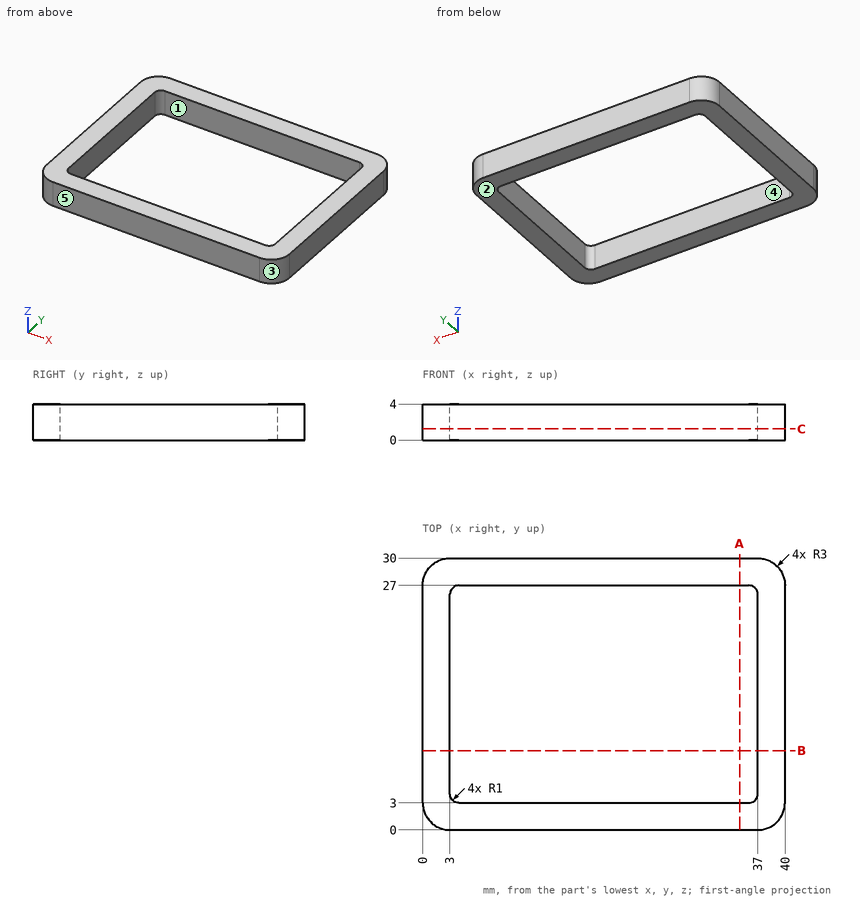
Geometry check sheet. Reference: drawing and pictorial views, mm from the part's lowest x, y, z. A direction names the side the tool comes from. Round coordinates to 2 decimals unless told otherwise and drop trailing zeros. Loops run counter-clockwise (first coordinate to the right, second up) from the corner with the lowest first, then second, coordinate; pieces in that order, holes last. Notation, with made-up numbers: (47.5, 12) -> (62.5, 12) arc R18 ccw to (62.5, 44) -> close; hole circle Ø6 at (58, 2.5). An arc over 180 degrees is marked (long way). Answer as a JSON object with one key per item and string values. Group by question number.
Item 1: Release check for a two-part mould opening along Y. For the marked faces 1, 2 and 3 record: pulls with the +Y half, pulls with the -Y half, needs draft (parallel to the pull), parting line crosses it, or undercut.
Item 2: Thickness scan on line 1 along X through (y, z) = (5.75, 2.5); line 2 along Y through (x, z) = (21, 3.85); line 3 along X through (y, z) = (26.75, 2.2). Record the ranges inside material, lowest first.
Item 3: Cross-section at B-B, the plane y = 8.75. Record the cut outline in (x, z), plus the area to 3 significant figures.
Item 4: Cross-section at C-C, the plane z = 1.25. Record the cut outline in (x, y), plus the area to 3 significant figures.
Item 5: Set-up check for the marked faces 4 and 5: record each of +Z, -Z, +X, -X, +Y, -Y from which the full face is reachable in a straight line by a thin tool's end or side.
Item 6: Cross-section at A-A, the plane x = 35. Record the cut outline in (y, z), plus the area to 3 significant figures.
Determined:
{
 "1": {"face 1": "undercut", "face 2": "needs draft", "face 3": "pulls with the -Y half"},
 "2": {"line 1": "x = 0 to 3, 37 to 40", "line 2": "y = 0 to 3, 27 to 30", "line 3": "x = 0 to 3.34, 36.66 to 40"},
 "3": {"outline": "(0, 0) -> (3, 0) -> (3, 4) -> (0, 4) -> close; (37, 0) -> (40, 0) -> (40, 4) -> (37, 4) -> close", "area": "24.0 mm²"},
 "4": {"outline": "(0, 3) arc R3 ccw to (3, 0) -> (37, 0) arc R3 ccw to (40, 3) -> (40, 27) arc R3 ccw to (37, 30) -> (3, 30) arc R3 ccw to (0, 27) -> close; hole (3, 4) arc R1 ccw to (4, 3) -> (36, 3) arc R1 ccw to (37, 4) -> (37, 26) arc R1 ccw to (36, 27) -> (4, 27) arc R1 ccw to (3, 26) -> close", "area": "377 mm²"},
 "5": {"face 4": "+Z, -Z", "face 5": "+Z, -Z, +X, -X, -Y"},
 "6": {"outline": "(0, 0) -> (3, 0) -> (3, 4) -> (0, 4) -> close; (27, 0) -> (30, 0) -> (30, 4) -> (27, 4) -> close", "area": "24.0 mm²"}
}
